Read the model definition and answer for the solid it produces. Units are mm, in the model's axes. A direction names the side the tool comes from. Coordinates: 2 decimals unless noted, no trailing zeros. Order: outer loops, then holes, each group sorted by start corner. A loop starts at its lowest first (then second) coordinate and runs counter-clockwise, first axis right, second up.
```python
from build123d import *
from build123d.topology import SkipClean

# Parameters (mm, degrees)
SKETCH2_W           = 108
SKETCH2_H           = 72
BOSS_EXTRUDE1_DEPTH = 20.64
SHELL1_T            = 5
SKETCH3_W           = 118
SKETCH3_H           = 82
CUT_EXTRUDE1_DEPTH  = 3
FILLET1_R           = 10
BOSS_EXTRUDE2_DEPTH = 6.985
CUT_EXTRUDE4_DEPTH  = 6.35
CUT_EXTRUDE2_DEPTH  = 1.875
SKETCH14_W          = 10.16
SKETCH14_H          = 63.5
SKETCH14_R          = 3.02514
BOSS_EXTRUDE5_DEPTH = 6.35


with BuildPart() as part:
    # Sketch2 → Boss-Extrude1 (new body)
    with BuildSketch(Plane.XY):
        Rectangle(SKETCH2_W, SKETCH2_H)
    extrude(amount=BOSS_EXTRUDE1_DEPTH)

    # Shell1
    shell1_openings = [part.faces().sort_by_distance(p)[0] for p in [
        (0, 0, 20.64),
    ]]
    offset(amount=SHELL1_T, openings=shell1_openings, kind=Kind.INTERSECTION)

    # Sketch3 → Cut-Extrude1 (cut)
    with BuildSketch(Plane(origin=(0, 0, -5), x_dir=(-1, 0, 0), z_dir=(0, 0, -1))):
        Rectangle(SKETCH3_W, SKETCH3_H)
    extrude(amount=-CUT_EXTRUDE1_DEPTH, mode=Mode.SUBTRACT)

    # Fillet1
    fillet1_edges = [part.edges().sort_by_distance(p)[0] for p in [
        (54, -36, 10.32),
        (54, 36, 10.32),
        (-54, 36, 10.32),
        (-54, -36, 10.32),
    ]]
    fillet(fillet1_edges, radius=FILLET1_R)

    # Sketch6 → Boss-Extrude2 (add)
    with BuildSketch(Plane.XY.offset(20.64)):
        with BuildLine():
            Line((59, -41), (60.27, -41))
            ThreePointArc((60.27, -41), (65.732714697, -34.86066586), (59, -30.148635688))
            Line((59, -30.148635688), (59, -41))
        make_face()
        with BuildLine():
            ThreePointArc((59, 30.148635688), (65.77, 35.5), (59, 40.851364312))
            Line((59, 40.851364312), (59, 30.148635688))
        make_face()
        with BuildLine():
            ThreePointArc((-59, -30.148635688), (-65.77, -35.5), (-59, -40.851364312))
            Line((-59, -40.851364312), (-59, -30.148635688))
        make_face()
        with BuildLine():
            ThreePointArc((-59, 40.851364312), (-65.77, 35.5), (-59, 30.148635688))
            Line((-59, 30.148635688), (-59, 40.851364312))
        make_face()
    boss_extrude2 = extrude(amount=-BOSS_EXTRUDE2_DEPTH)

    # Sketch6_4 → Cut-Extrude4 (cut)
    with BuildSketch(Plane.XY.offset(20.64)):
        with BuildLine():
            Line((59, 38.245491759), (59, 32.754508241))
            ThreePointArc((59, 32.754508241), (61.899244457, 32.951238046), (63.295, 35.5))
            ThreePointArc((63.295, 35.5), (61.899244457, 38.048761954), (59, 38.245491759))
        make_face()
        with BuildLine():
            ThreePointArc((59, 38.245491759), (57.245, 35.5), (59, 32.754508241))
            Line((59, 32.754508241), (59, 38.245491759))
        make_face()
        with BuildLine():
            Line((59, -38.245491759), (59, -32.754508241))
            ThreePointArc((59, -32.754508241), (57.245, -35.5), (59, -38.245491759))
        make_face()
        with BuildLine():
            ThreePointArc((63.295, -35.5), (61.899244457, -32.951238046), (59, -32.754508241))
            Line((59, -32.754508241), (59, -38.245491759))
            ThreePointArc((59, -38.245491759), (61.899244457, -38.048761954), (63.295, -35.5))
        make_face()
        with BuildLine():
            ThreePointArc((-59, -38.245491759), (-57.721238046, -37.129244457), (-57.245, -35.5))
            ThreePointArc((-57.245, -35.5), (-57.721238046, -33.870755543), (-59, -32.754508241))
            Line((-59, -32.754508241), (-59, -38.245491759))
        make_face()
        with BuildLine():
            Line((-59, -38.245491759), (-59, -32.754508241))
            ThreePointArc((-59, -32.754508241), (-63.295, -35.5), (-59, -38.245491759))
        make_face()
        with BuildLine():
            Line((-59, 38.245491759), (-59, 32.754508241))
            ThreePointArc((-59, 32.754508241), (-57.721238046, 33.870755543), (-57.245, 35.5))
            ThreePointArc((-57.245, 35.5), (-57.721238046, 37.129244457), (-59, 38.245491759))
        make_face()
        with BuildLine():
            ThreePointArc((-59, 38.245491759), (-63.295, 35.5), (-59, 32.754508241))
            Line((-59, 32.754508241), (-59, 38.245491759))
        make_face()
    cut_extrude4 = extrude(amount=-CUT_EXTRUDE4_DEPTH, mode=Mode.SUBTRACT)

    # Mirror5: Boss-Extrude2, Cut-Extrude4 across plane
    with SkipClean():  # the faces are left unmerged after this step: merging them gives an invalid solid
        add(boss_extrude2.mirror(Plane(origin=(0, 0, 0), x_dir=(0, 0, 1), z_dir=(1, 0, 0))))
        add(cut_extrude4.mirror(Plane(origin=(0, 0, 0), x_dir=(0, 0, 1), z_dir=(1, 0, 0))), mode=Mode.SUBTRACT)

    # Sketch5 → Cut-Extrude2 (cut)
    with SkipClean():  # the faces are left unmerged after this step: merging them gives an invalid solid
        with BuildSketch(Plane.XY.offset(20.64)):
            with BuildLine():
                Line((46.071067812, -39.11), (-46.071067812, -39.11))
                ThreePointArc((-46.071067812, -39.11), (-54.050767838, -35.804700026), (-57.356067812, -27.825))
                Line((-57.356067812, -27.825), (-57.356067812, 28.071067812))
                ThreePointArc((-57.356067812, 28.071067812), (-54.050767838, 36.050767838), (-46.071067812, 39.356067812))
                Line((-46.071067812, 39.356067812), (46.071067812, 39.356067812))
                ThreePointArc((46.071067812, 39.356067812), (54.050767838, 36.050767838), (57.356067812, 28.071067812))
                Line((57.356067812, 28.071067812), (57.356067812, -27.825))
                ThreePointArc((57.356067812, -27.825), (54.050767838, -35.804700026), (46.071067812, -39.11))
            make_face()
            with BuildLine():
                Line((46.071067812, -36.54), (-46.071067812, -36.54))
                ThreePointArc((-46.071067812, -36.54), (-52.23350341, -33.987435598), (-54.786067812, -27.825))
                Line((-54.786067812, -27.825), (-54.786067812, 28.071067812))
                ThreePointArc((-54.786067812, 28.071067812), (-52.23350341, 34.23350341), (-46.071067812, 36.786067812))
                Line((-46.071067812, 36.786067812), (46.071067812, 36.786067812))
                ThreePointArc((46.071067812, 36.786067812), (52.23350341, 34.23350341), (54.786067812, 28.071067812))
                Line((54.786067812, 28.071067812), (54.786067812, -27.825))
                ThreePointArc((54.786067812, -27.825), (52.23350341, -33.987435598), (46.071067812, -36.54))
            make_face(mode=Mode.SUBTRACT)
        extrude(amount=-CUT_EXTRUDE2_DEPTH, mode=Mode.SUBTRACT)

    # Sketch14 → Boss-Extrude5 (add)
    with SkipClean():  # the faces are left unmerged after this step: merging them gives an invalid solid
        with BuildSketch(Plane(origin=(59, 0, 0), x_dir=(0, 0, -1), z_dir=(1, 0, 0))):
            with Locations((-6.035, -9.25)):
                Rectangle(SKETCH14_W, SKETCH14_H)
            with Locations(Location((-6.035, 8.04994, 0), (0, 0, 90))):
                Circle(SKETCH14_R, mode=Mode.SUBTRACT)
            with Locations(Location((-6.035, -21.95, 0), (0, 0, 90))):
                Circle(SKETCH14_R, mode=Mode.SUBTRACT)
        boss_extrude5 = extrude(amount=BOSS_EXTRUDE5_DEPTH)

    # Mirror6: Boss-Extrude5 across plane
    with SkipClean():  # the faces are left unmerged after this step: merging them gives an invalid solid
        add(boss_extrude5.mirror(Plane(origin=(0, 0, 0), x_dir=(0, 0, 1), z_dir=(1, 0, 0))))


solid = part.part
```
1) Which of the six approach directions +Z, -Z, +X, -X, +Y, -Y give full straight-line access (tool end or side, diameter ignored) to faces 5 (the flat face through (-62, 36, 13.655)), 6 (the flat face through (-62, 22.5, 6)), 7 (the cylindrical face through (-62.131, 10.844, 4.876)), 8 (the cylindrical face through (62.131, 10.844, 4.876)), 9 (the cylindrical face through (-52.17, -34.05, 19.72))?
A:
face 5: -Z, -X, +Y, -Y
face 6: +Z, -Z, -X, +Y
face 7: -X
face 8: +X
face 9: +Z
2) A cutting plane is placed at A-A, the plane x = -11. Determine the outline of the cut face in (y, z) (3 decimals), and give its area (3 significant figures).
A:
outline: (-41, -2) - (41, -2) - (41, 20.64) - (39.356, 20.64) - (39.356, 18.765) - (36.786, 18.765) - (36.786, 20.64) - (36, 20.64) - (36, 0) - (-36, 0) - (-36, 20.64) - (-36.54, 20.64) - (-36.54, 18.765) - (-39.11, 18.765) - (-39.11, 20.64) - (-41, 20.64) - close
area: 361 mm2
3) Flat-ended cylindrical pins translate along their axes: pin 1 Ø5 at (y, z) = (8.05, 6.04) entering from +X; pin 2 Ø7.5 at (x, y) = (63, -35.5) entering from -Z (3 decimals); pin 3 Ø10 at (x, y) = (51.5, 31.5) entering from +Z; pin 4 Ø7 at (y, z) = (-1, 12) entering from -X. Find the tip coordinate at first contact, or state that the pin passes through.
A:
pin 1: stops at x = 59
pin 2: stops at z = 0.955
pin 3: stops at z = 20.64
pin 4: stops at x = -65.35
4) Determine the mould class of faces 1 (the flat face through (65.35, -9, 6)), 2 (the flat face through (1, -41, 9)), 3 (the flat face through (-59, -22, 6)), 4 (the cylindrical face through (54, 36.1, 19.7)) for opening direction X: pulls with the +X half, pulls with the -X half, needs draft (parallel to the pull), parting line crosses it, or undercut.
A:
face 1: pulls with the +X half
face 2: needs draft
face 3: pulls with the -X half
face 4: undercut
5) Straight lines are drawn through the part: line 1 (Y direction, x = 60.27, z = 19) (3 decimals); line 2 (X direction, y = -9.5, z = 10.25); line 3 (Y direction, x = -7.5, z = 3.5). For each, find the intervals that lie inside material, in ascending order.
A:
line 1: y = -41 to -38.525, -32.475 to -30, 30 to 32.475, 38.525 to 41
line 2: x = -65.35 to -54, 54 to 65.35
line 3: y = -41 to -36, 36 to 41
6) A cutting plane is placed at D-D, the plane x = 47.5. Determine the outline of the cut face in (y, z) (1 decimal), and give its area (3 significant figures).
A:
outline: (-41, -2) - (41, -2) - (41, 20.6) - (39.3, 20.6) - (39.3, 18.8) - (36.7, 18.8) - (36.7, 20.6) - (35.4, 20.6) - (35.4, 0) - (-35.4, 0) - (-35.4, 20.6) - (-36.4, 20.6) - (-36.4, 18.8) - (-39, 18.8) - (-39, 20.6) - (-41, 20.6) - close
area: 387 mm2
7) A cutting plane is placed at B-B, the plane x = -60.27. Determine the outline of the cut face in (y, z) (3 decimals).
A:
outline: (-41, 0.955) - (22.5, 0.955) - (22.5, 11.115) - (-41, 11.115) - close; (-41, 13.655) - (-30, 13.655) - (-30, 20.64) - (-32.475, 20.64) - (-32.475, 14.29) - (-38.525, 14.29) - (-38.525, 20.64) - (-41, 20.64) - close; (30, 13.655) - (41, 13.655) - (41, 20.64) - (38.525, 20.64) - (38.525, 14.29) - (32.475, 14.29) - (32.475, 20.64) - (30, 20.64) - close; hole circle Ø6.05 at (-21.95, 6.035); hole circle Ø6.05 at (8.05, 6.035)
